Geometry check sheet. Reference: the model listing, model coordinates, mm. Round coordinates to 2 decimals unless told otherwise and drop trailing zeros. Write each loop counter-clockwise with the first axis right and the second up, starting at its lowest first coordinate (ties: lowest second). Pieces come first, ordered by that corner, then holes.
Item 1: Cross-section at A-A (y = -30.48). Enter the section's corners in (x, z), then the cut area to 3 significant figures.
Item 2: Depth check by flat-ended pin: P1, Ø0.7, axis at x = 78.74, y = -17.78, coming from the -Z side. Enter the tip coordinate at first touch or a pass-through.
Item 3: Scan lines: probe 1 along Y at (x, z) = (83.82, 0.9); probe 2 along Y at (x, z) = (52.74, 0.65); probe 3 along Y at (x, z) = (38.1, 0.45). Record each from-to range of solid material in increasing order.
from build123d import *

# Parameters (mm, degrees)
SKETCH1_W                 = 88.9
SKETCH1_H                 = 45.72
BOARD_SHAPE_EXTRUDE_DEPTH = 1.5748
SKETCH2_R                 = 0.55
MMC_MOUNT_HOLE_CUT_DEPTH  = 1.5748
SKETCH4_R                 = 0.508
HFBR_ANCHOR_HOLES_DEPTH   = 1.5748
SKETCH5_R                 = 2.032
CUT_EXTRUDE3_DEPTH        = 1.5748


with BuildPart() as part:
    # Sketch1 → board shape -extrude (new body)
    with BuildSketch(Plane.XY):
        with Locations((44.45, -22.86)):
            Rectangle(SKETCH1_W, SKETCH1_H)
    extrude(amount=BOARD_SHAPE_EXTRUDE_DEPTH)

    # Sketch2 → mmc mount hole - cut (cut)
    with BuildSketch(Plane.XY.offset(1.5748)):
        with Locations((52.74, -17.78)):
            Circle(SKETCH2_R)
        with Locations((78.74, -17.78)):
            Circle(SKETCH2_R)
    extrude(amount=-MMC_MOUNT_HOLE_CUT_DEPTH, mode=Mode.SUBTRACT)

    # Sketch4 → HFBR anchor holes (cut)
    with BuildSketch(Plane.XY.offset(1.5748)):
        with Locations((20.32, -42.164)):
            Circle(SKETCH4_R)
        with Locations((27.94, -42.164)):
            Circle(SKETCH4_R)
        with Locations((30.48, -42.164)):
            Circle(SKETCH4_R)
        with Locations((38.1, -42.164)):
            Circle(SKETCH4_R)
    extrude(amount=-HFBR_ANCHOR_HOLES_DEPTH, mode=Mode.SUBTRACT)

    # Sketch5 → Cut-Extrude3 (cut)
    with BuildSketch(Plane.XY.offset(1.5748)):
        with Locations((83.82, -30.48)):
            Circle(SKETCH5_R)
        with Locations((83.82, -12.7)):
            Circle(SKETCH5_R)
        with Locations((19.304, -19.812)):
            Circle(SKETCH5_R)
    extrude(amount=-CUT_EXTRUDE3_DEPTH, mode=Mode.SUBTRACT)


solid = part.part
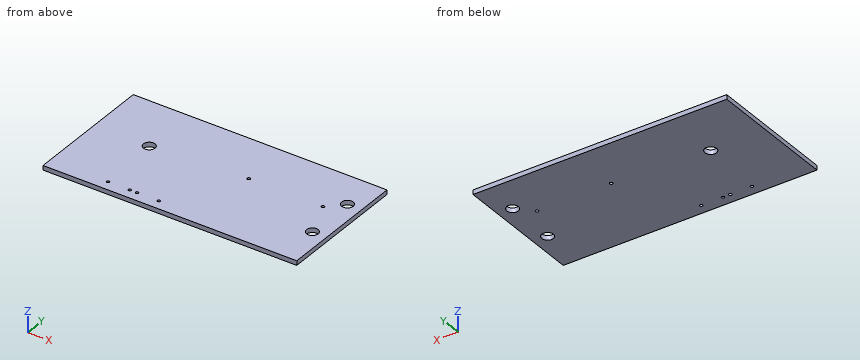
Resolved:
1. outline: (0, 0) - (81.79, 0) - (81.79, 1.57) - (0, 1.57) - close; (85.85, 0) - (88.9, 0) - (88.9, 1.57) - (85.85, 1.57) - close
1. area: 134 mm2
2. P1: passes through
3. probe 1: y = -45.72 to -32.51, -28.45 to -14.73, -10.67 to 0
3. probe 2: y = -45.72 to -18.33, -17.23 to 0
3. probe 3: y = -45.72 to -42.67, -41.66 to 0
